Read the model definition and answer for the solid it produces. Units are mm, in the model's axes. A direction names the side the tool comes from. Give positions to 0.01 mm unless a question says otherwise; leave off trailing zeros. Loops run counter-clockwise (first coordinate to the right, second up) from the corner with the lowest first, then second, coordinate; pieces in that order, holes last. Notation, with made-up numbers: (87, 41.5) -> (96, 41.5) arc R20 ccw to (96, 46.5) -> close; hole circle Ø6 at (80, -14). An arc over 180 degrees is marked (long way). Answer as CSV lines item,"result". Start each with the question number.
```python
from build123d import *

# Parameters (mm, degrees)
BOSS_EXTRUDE1_DEPTH = 3
BOSS_EXTRUDE2_DEPTH = 7
SKETCH4_R           = 6.5
BOSS_EXTRUDE3_DEPTH = 4
FILLET1_R           = 2
FILLET2_R           = 1
SKETCH5_R           = 2.25
CUT_EXTRUDE1_DEPTH  = 32.180923655


with BuildPart() as part:
    # Sketch1 → Revolve1 (revolve)
    with BuildSketch(Plane.XY, mode=Mode.PRIVATE) as revolve1_sk:
        Polygon((11, 0), (11, 6), (0, 6), (0, 7), (-7, 7), (-7, 0), align=None)
    revolve(revolve1_sk.sketch.rotate(Axis((-13.395348837, 0, 0), (1, 0, 0)), 90), axis=Axis((-13.395348837, 0, 0), (1, 0, 0)))

    # Sketch2 → Boss-Extrude1 (add)
    with BuildSketch(Plane(origin=(0, 0, 0), x_dir=(0, 0, -1), z_dir=(1, 0, 0))):
        Polygon((4.330127019, -7.5), (8.660254038, 0), (4.330127019, 7.5), (-4.330127019, 7.5), (-8.660254038, 0), (-4.330127019, -7.5), align=None)
    extrude(amount=BOSS_EXTRUDE1_DEPTH)

    # Sketch3 → Boss-Extrude2 (add)
    with BuildSketch(Plane.ZY.offset(7)):
        Polygon((4.330127019, -7.5), (8.660254038, 0), (4.330127019, 7.5), (-4.330127019, 7.5), (-8.660254038, 0), (-4.330127019, -7.5), align=None)
    extrude(amount=BOSS_EXTRUDE2_DEPTH)

    # Sketch4 → Boss-Extrude3 (add)
    with BuildSketch(Plane.ZY.offset(14)):
        Circle(SKETCH4_R)
    extrude(amount=BOSS_EXTRUDE3_DEPTH)

    # Fillet1
    fillet1_edges = [part.edges().sort_by_distance(p)[0] for p in [
        (-18, 0, -6.5),
    ]]
    fillet(fillet1_edges, radius=FILLET1_R)

    # Fillet2
    fillet2_edges = [part.edges().sort_by_distance(p)[0] for p in [
        (-14, -7.5, 0),
        (-14, -3.75, 6.495190528),
        (-14, 3.75, 6.495190528),
        (-14, 7.5, 0),
        (-14, 3.75, -6.495190528),
        (-14, -3.75, -6.495190528),
    ]]
    fillet(fillet2_edges, radius=FILLET2_R - 0.0001)  # a hair under: the kernel refuses the full size

    # Sketch5 → Cut-Extrude1 (cut, through all)
    with BuildSketch(Plane.ZY.offset(18)):
        Circle(SKETCH5_R)
    extrude(amount=-CUT_EXTRUDE1_DEPTH, mode=Mode.SUBTRACT)


solid = part.part
```
(1) A tool of negligible diameter and unlimited length cuts with its end or side. For faces 4 (the face through (-14.986, -3.955, -5.158)), 5 (the face through (1.479, -3.698, 6.526)), 6 (the face through (0, -3.3, -6.4)), from which of +Z, -Z, +X, -X, +Y, -Y can it reach the whole face along a straight path? Write none if from no direction.
(2) Find section C-C on x = -4.5. Write down the section's boundary in (y, z).
(3) The mould has two halves that part along X. Classify faces 1 (the face through (-7, -3.3, 6.4)), 2 (the face through (-13.715, -3.652, -6.204)), 3 (the face through (-9.958, -3.802, 6.465)): pulls with the +X half, pulls with the -X half, needs draft (parallel to the pull), parting line crosses it, or undercut.
(4) Find the intervals of material crossed by line 1 along Y through (x, z) = (-10, 0); line 2 along Y through (x, z) = (5, 0); line 3 along X through (y, z) = (-5.75, -4.25), in increasing order. Write a range as from..to.
(5) Find section D-D on x = -15. Write down the section's boundary in (y, z), then the cut area to 3 significant figures.
(6) Find section A-A on x = -8. Write down the section's boundary in (y, z).
(7) Each of these flat-tipped pins is pushed along its axis until it touches: P1, Ø1.5, axis at x = 6, z = 0, coming from the -Y side; P2, Ø1.5, axis at x = 1, y = -2.5, coming from the -Z side. Where does it stop, or does it pass through?
Answer block:
1,face 4,"-X"
1,face 5,"+Z, +X, -X, -Y"
1,face 6,"none"
2,outline,"circle Ø14 at (0, 0); hole circle Ø4.5 at (0, 0)"
3,face 1,"undercut"
3,face 2,"pulls with the -X half"
3,face 3,"needs draft"
4,line 1,"y = -7.5..-2.25, 2.25..7.5"
4,line 2,"y = -6..-2.25, 2.25..6"
4,line 3,"x = -14..-7, 0..3"
5,outline,"circle Ø13 at (0, 0); hole circle Ø4.5 at (0, 0)"
5,area,"117 mm2"
6,outline,"(-7.5, -4.33) -> (0, -8.66) -> (7.5, -4.33) -> (7.5, 4.33) -> (0, 8.66) -> (-7.5, 4.33) -> close; hole circle Ø4.5 at (0, 0)"
7,P1,"stops at y = -6"
7,P2,"stops at z = -7.65"
